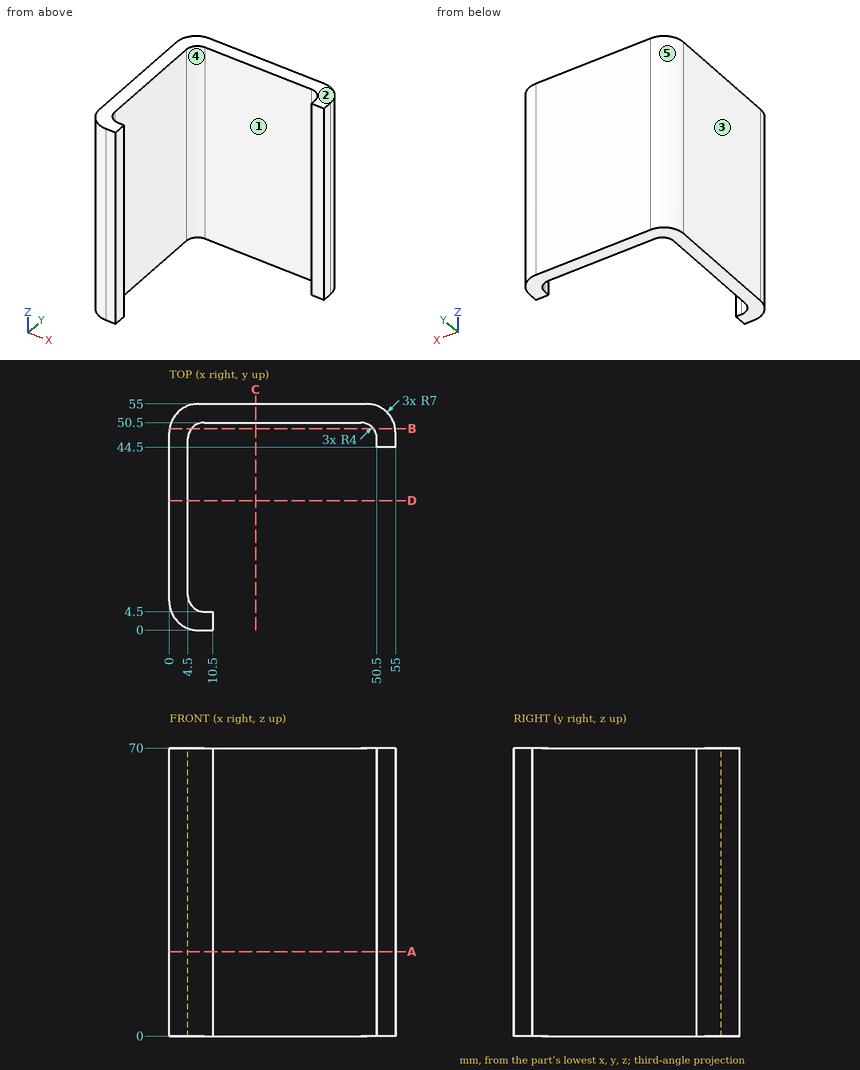
The figure shows three views and two pictorial views of one solid part (mm, origin at its lowest corner). Answer the questions. A direction names the side the tool comes from. Give positions to 0.01 mm unless a question says otherwise; leave off trailing zeros. Loops run counter-clockwise (first coordinate to the right, second up) from the corner with the lowest first, then second, coordinate; pieces in that order, holes last. Notation, with made-up numbers: (-35.75, 84.5) -> (-11.75, 84.5) arc R13 ccw to (-11.75, 102.5) -> close; hole circle Ø11 at (-26.75, 24.5). An arc over 180 degrees is marked (long way). Use a Markdown table: item, result. Add a question column.
1. Section B-B on y = 49 is taken. Determine the outline of the cut face in (x, z), and give its area (3 significant figures).
2. Section D-D on y = 31.5 is taken. Determine the outline of the cut face in (x, z).
3. Flat-ended cylindrical pins translate along their axes: pin 1 Ø1 at (x, z) = (22, 51.5) entering from -Y; pin 2 Ø5 at (y, z) = (2.5, 30) entering from +X; pin 3 Ø1.3 at (x, z) = (52.5, 51.5) entering from -Y. Find the tip coordinate at first contact, or state that the pin passes through.
4. For the marked faces 4 and 5, determine the directions among +Z, -Z, +X, -X, +Y, -Y from which every point of the face is accessible in a straight line to the end or side of a thin tool.
5. Section A-A on z = 20.5 is taken. Determine the outline of the cut face in (x, y).
6. Determine the mould class of the marked faces 1, 2 and 3 for opening direction X: released by +X, released by -X, zero draft, split by the parting line, or undercut.
7. Find the intervals of material crossed by probe 1 along X at (y, z) = (26.5, 34.5); probe 2 along Y at (x, z) = (43.5, 57.5); probe 3 along Y at (x, z) = (8, 57.5), in increasing order.
8. Section C-C on x = 21 is taken. Determine the outline of the cut face in (y, z), and give its area (3 significant figures).
Results below:
| question | item | result |
|---|---|---|
| 1 | outline | (0.07, 0) -> (5.38, 0) -> (5.38, 70) -> (0.07, 70) -> close; (49.62, 0) -> (54.93, 0) -> (54.93, 70) -> (49.62, 70) -> close |
| 1 | area | 743 mm^2 |
| 2 | outline | (0, 0) -> (4.5, 0) -> (4.5, 70) -> (0, 70) -> close |
| 3 | pin 1 | stops at y = 50.5 |
| 3 | pin 2 | stops at x = 10.5 |
| 3 | pin 3 | stops at y = 44.5 |
| 4 | face 4 | +Z, -Z |
| 4 | face 5 | +Z, -Z, -X, +Y |
| 5 | outline | (0, 7) arc R7 ccw to (7, 0) -> (10.5, 0) -> (10.5, 4.5) -> (8.5, 4.5) arc R4 cw to (4.5, 8.5) -> (4.5, 46.5) arc R4 cw to (8.5, 50.5) -> (46.5, 50.5) arc R4 cw to (50.5, 46.5) -> (50.5, 44.5) -> (55, 44.5) -> (55, 48) arc R7 ccw to (48, 55) -> (7, 55) arc R7 ccw to (0, 48) -> close |
| 6 | face 1 | undercut |
| 6 | face 2 | zero draft |
| 6 | face 3 | released by -X |
| 7 | probe 1 | x = 0 to 4.5 |
| 7 | probe 2 | y = 50.5 to 55 |
| 7 | probe 3 | y = 0 to 4.53, 50.47 to 55 |
| 8 | outline | (50.5, 0) -> (55, 0) -> (55, 70) -> (50.5, 70) -> close |
| 8 | area | 315 mm^2 |
